Study the drawing (mm; zero at the part's minimum x, y, z) and answer. Coordinates: 2 decimals unless noted, no trailing zeros. Loops run counter-clockwise (first coordinate to the right, second up) from the corner with the lowest first, then second, coordinate; pieces in that order, holes last.
Q1. Straight lines are drawn through the part: line 1 (Y direction, x = 19, z = 10.25); line 2 (Z direction, x = 19.55, y = 66.5); line 3 (Z direction, x = 14.5, y = 49). For each, find the intervals that lie inside material, in ascending order.
Q2. Section D-D (z = 5.5) is taken. Give the vertices of the cut face in (x, y).
Q3. Section B-B (x = 8) is taken. Give the vertices of the cut face in (y, z) (1 decimal).
Q4. Flat-ended cylindrical pins translate along their axes: P1, Ø1, axis at y = 41.5, z = 17, coming from the -X side; P2, Ø6, axis at y = 22, z = 5, coming from the +X side; P3, Ø0.7, axis at x = 4, y = 40, coming from the +Z side. Find the tip coordinate at first contact, or state that the pin passes through.
Q5. Section C-C (y = 66.5) is taken. Give the vertices of the cut face in (x, z).
Q6. Section A-A (z = 11) is taken. Give the vertices of the cut face in (x, y), then the cut area to 3 significant figures.
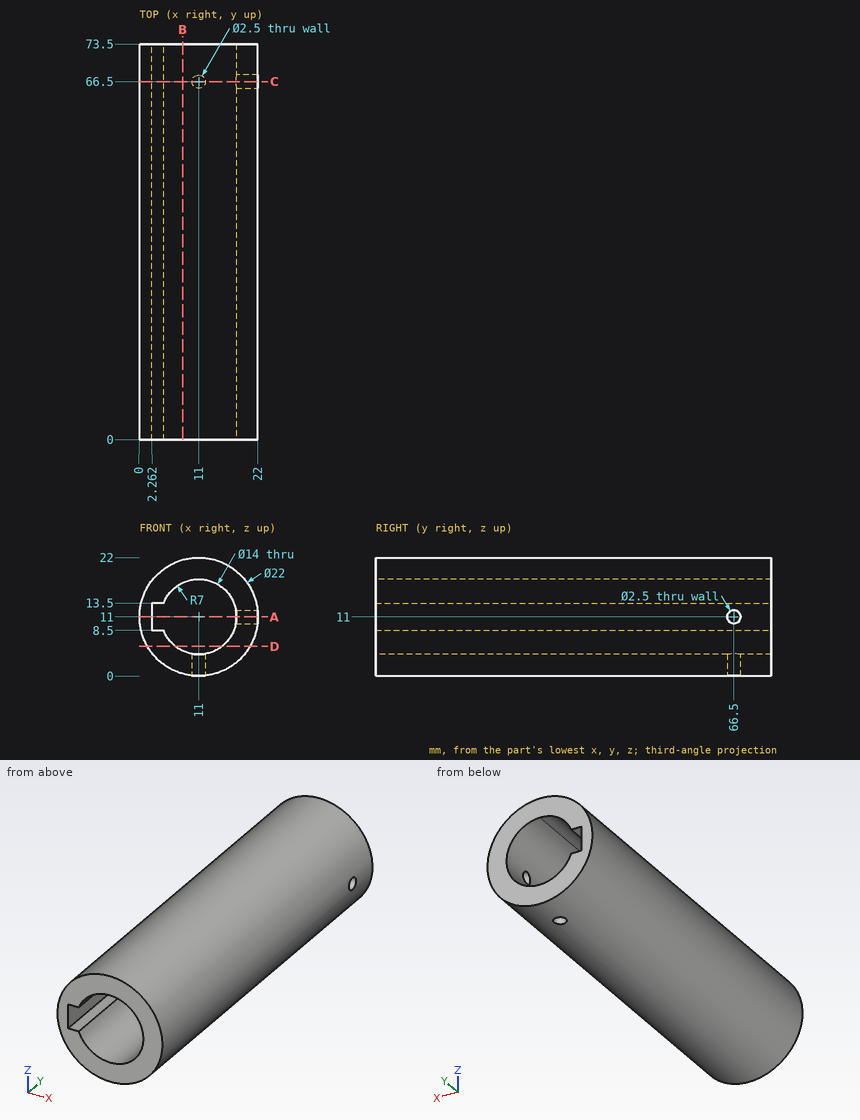
Numbers:
1. line 1: y = 0 to 65.5, 67.5 to 73.5
1. line 2: z = 4.08 to 9.75, 12.25 to 17.92
1. line 3: z = 0.57 to 4.94, 17.06 to 21.43
2. outline: (1.47, 0) - (6.67, 0) - (6.67, 73.5) - (1.47, 73.5) - close; (15.33, 0) - (20.53, 0) - (20.53, 73.5) - (15.33, 73.5) - close
3. outline: (0, 0.4) - (73.5, 0.4) - (73.5, 4.7) - (0, 4.7) - close; (0, 17.3) - (73.5, 17.3) - (73.5, 21.6) - (0, 21.6) - close
4. P1: stops at x = 1.47
4. P2: stops at x = 21.58
4. P3: stops at z = 19.76
5. outline: (2.26, 8.5) - (2.26, 13.5) - (4.46, 13.5) arc R7 cw to (17.89, 12.25) - (21.93, 12.25) arc R11 ccw (long way) to (9.75, 0.07) - (9.75, 4.11) arc R7 cw to (4.46, 8.5) - close; (12.25, 0.07) arc R11 ccw to (21.93, 9.75) - (17.89, 9.75) arc R7 cw to (12.25, 4.11) - close
6. outline: (0, 0) - (2.26, 0) - (2.26, 73.5) - (0, 73.5) - close; (18, 0) - (22, 0) - (22, 65.25) - (18, 65.25) - close; (18, 67.75) - (22, 67.75) - (22, 73.5) - (18, 73.5) - close
6. area: 450 mm2
